```python
from build123d import *

# Parameters (mm, degrees)
SKETCH1_R                = 24
BOSS_EXTRUDE1_DEPTH      = 10
SKETCH2_R                = 14
BOSS_EXTRUDE2_DEPTH      = 34
CUT_EXTRUDE1_REACH       = 46
SKETCH3_W                = 82.684433326
SKETCH3_H                = 23.530230521
SKETCH3_W_2              = 72.226300178
SKETCH3_H_2              = 23.293039824
CUT_EXTRUDE2_REACH       = 46
SKETCH4_R                = 8
SKETCH7_R                = 2.75
CUT_EXTRUDE3_DEPTH       = 10
CHAMFER1_SIZE            = 0.5
CHAMFER1_OF_MIRROR1_SIZE = 0.5
CHAMFER2_SIZE            = 0.5


with BuildPart() as part:
    # Sketch1 → Boss-Extrude1 (new body)
    with BuildSketch(Plane.XY):
        Circle(SKETCH1_R)
    extrude(amount=BOSS_EXTRUDE1_DEPTH)

    # Sketch2 → Boss-Extrude2 (add)
    with BuildSketch(Plane(origin=(0, 0, 0), x_dir=(-1, 0, 0), z_dir=(0, 0, -1))):
        Circle(SKETCH2_R)
    extrude(amount=BOSS_EXTRUDE2_DEPTH)

    # Sketch3 → Cut-Extrude1 (cut, up to next)
    with BuildSketch(Plane.XY.offset(10), mode=Mode.PRIVATE) as cut_extrude1_sk1:
        with Locations((-2.888944578, 31.765115261)):
            Rectangle(SKETCH3_W, SKETCH3_H)
    cut_extrude1_tool1 = extrude(cut_extrude1_sk1.sketch, amount=-CUT_EXTRUDE1_REACH, mode=Mode.PRIVATE) & part.part
    add(cut_extrude1_tool1.solids().sort_by_distance((-2.888945, 31.765115, 10))[0], mode=Mode.SUBTRACT)
    # Sketch3 → Cut-Extrude1 (cut, up to next)
    with BuildSketch(Plane.XY.offset(10), mode=Mode.PRIVATE) as cut_extrude1_sk2:
        with Locations((2.340121996, -31.646519912)):
            Rectangle(SKETCH3_W_2, SKETCH3_H_2)
    cut_extrude1_tool2 = extrude(cut_extrude1_sk2.sketch, amount=-CUT_EXTRUDE1_REACH, mode=Mode.PRIVATE) & part.part
    add(cut_extrude1_tool2.solids().sort_by_distance((2.340122, -31.64652, 10))[0], mode=Mode.SUBTRACT)

    # Sketch4 → Cut-Extrude2 (cut, up to next)
    with BuildSketch(Plane(origin=(0, 0, -34), x_dir=(-1, 0, 0), z_dir=(0, 0, -1)), mode=Mode.PRIVATE) as cut_extrude2_sk1:
        Circle(SKETCH4_R)
    cut_extrude2_tool1 = extrude(cut_extrude2_sk1.sketch, amount=-CUT_EXTRUDE2_REACH, mode=Mode.PRIVATE) & part.part
    add(cut_extrude2_tool1.solids().sort_by_distance((0, 0, -34))[0], mode=Mode.SUBTRACT)

    # Sketch7 → Cut-Extrude3 (cut)
    with BuildSketch(Plane.XY.offset(10)):
        with Locations((-13.435028843, 13.435028843)):
            Circle(SKETCH7_R)
        with Locations((-19, 0)):
            Circle(SKETCH7_R)
        with Locations((-13.435028843, -13.435028843)):
            Circle(SKETCH7_R)
    cut_extrude3 = extrude(amount=-CUT_EXTRUDE3_DEPTH, mode=Mode.SUBTRACT)

    # Chamfer1
    chamfer1_edges = [part.edges().sort_by_distance(p)[0] for p in [
        (-16.185028843, 13.435028843, 10),
        (-21.75, 0, 10),
        (-16.185028843, -13.435028843, 10),
    ]]
    chamfer(chamfer1_edges, length=CHAMFER1_SIZE)

    # Mirror1: Cut-Extrude3 across plane
    add(cut_extrude3.mirror(Plane(origin=(0, 0, 0), x_dir=(0, 0, 1), z_dir=(1, 0, 0))), mode=Mode.SUBTRACT)

    # Chamfer1 of Mirror1
    chamfer1_of_mirror1_edges = [part.edges().sort_by_distance(p)[0] for p in [
        (16.185028843, 13.435028843, 10),
        (21.75, 0, 10),
        (16.185028843, -13.435028843, 10),
    ]]
    chamfer(chamfer1_of_mirror1_edges, length=CHAMFER1_OF_MIRROR1_SIZE)

    # Chamfer2
    chamfer2_edges = [part.edges().sort_by_distance(p)[0] for p in [
        (-24, 0, 0),
        (24, 0, 10),
        (24, 0, 0),
        (14, 0, -34),
        (-24, 0, 10),
    ]]
    chamfer(chamfer2_edges, length=CHAMFER2_SIZE)


solid = part.part
```
Check sheet for the modelled part. Datum: model origin and axes. Units: mm. A direction names the side the tool comes from. Coordinates: 2 decimals unless noted, no trailing zeros. Order: outer loops, then holes, each group sorted by start corner. A loop starts at its lowest first (then second) coordinate and runs counter-clockwise, first axis right, second up. Notation, with made-up numbers: M 25.25,18 L 44.25,18 A19 cw 44.25,28 Z; hole C -25.75,83.25 d6. An arc over 180 degrees is marked long. Write each question's results on one line, items separated by ' | '. Start each with the question number.
1. Mould release check, pull along Y, two halves, no side actions. Record for faces 1 (the face through (-6, -6, -34)), 2 (the face through (-24, 0, 5)), 3 (the face through (15.462, -11.576, 4.816)): +Y half, -Y half, draft (parallel to the pull), parting line (faces both ways), or undercut.
2. Go/stop test with flat-tipped pins: P1, Ø1.5, axis at x = -12, z = -28.5, coming from the -Y side; P2, Ø4.5, axis at x = -19, y = 0, coming from the +Z side; P3, Ø5, axis at x = 7.5, z = -10, coming from the -Y side; P4, Ø9, axis at x = -13.44, y = 13.44, coming from the -Z side. Record where each tip stops, or that it passes through.
3. Access from +Z, -Z, +X, -X, +Y, -Y to the whole of each face (thin tool, end or side, straight path). Record for faces 4 (the face through (-21.747, 0.121, 4.816)), 5 (the face through (5, 14, 0)).
4. Cross-section at B-B on y = 0. State how many separate pieces and enclosed holes the cut face has, and give its area (3 significant figures).
5. Material ranges on probe 1 along Z at (x, y) = (21, 10.5); probe 2 along X at (y, z) = (-12, 4); probe 3 along Y at (x, z) = (-19, 3), recorded low to high.
6. Cross-section at C-C on z = -17. Record the cut outline in (x, y), and give its area (3 significant figures).
7. Cross-section at A-A on x = 0. Record the cut outline in (y, z).
Checks:
1) face 1: draft | face 2: parting line | face 3: undercut
2) P1: stops at y = -8.33 | P2: passes through | P3: stops at y = -13.08 | P4: stops at z = 0
3) face 4: +Z, -Z | face 5: -Z
4) separate pieces: 4 | enclosed holes: 0 | area: 617 mm²
5) probe 1: z = 0 to 10 | probe 2: x = -20.78 to -15.78, -11.09 to 11.09, 15.78 to 20.78 | probe 3: y = -14.66 to -2.75, 2.75 to 14.66
6) outline: C 0,0 d28; hole C 0,0 d16 | area: 415 mm²
7) outline: M -20,0 L -14,0 L -14,-33.5 L -13.5,-34 L -8,-34 L -8,10 L -20,10 Z; M 8,-34 L 13.5,-34 L 14,-33.5 L 14,0 L 20,0 L 20,10 L 8,10 Z
